Autodesk Fusion 360 part; units mm, degrees
sketch "Sketch1" plane through (0, 0, 0) normal (0, 1, 0) x (1, 0, 0)
  line L0 (0, 0) -> (-85, 0)
  line L1 (0, 0) -> (0, -98)
  line L2 (-85, 0) -> (-85, -20)
  line L3 (-85, -20) -> (-73, -20)
  line L4 (-73, -20) -> (-73, -68)
  line L5 (-73, -68) -> (-50, -98)
  line L6 (-50, -98) -> (0, -98)
  line L7 (50, -98) -> (0, -98)
  line L8 (73, -68) -> (50, -98)
  line L9 (73, -20) -> (73, -68)
  line L10 (85, -20) -> (73, -20)
  line L11 (85, 0) -> (85, -20)
  line L12 (0, 0) -> (85, 0)
  dimension "d1" = 85
  dimension "d2" = 20
  dimension "d3" = 12
  dimension "d4" = 48
  dimension "d5" = 98
  dimension "d6" = 50
extrude "Extrude1" add sketch "Sketch1" along normal blind 10
sketch "Sketch2" plane through (0, 10, 0) normal (0, 1, 0) x (-1, 0, 0)
  line L0 (85, 0) -> (85, 20)
  line L1 (85, 20) -> (73, 20)
  line L2 (73, 20) -> (73, 68)
  line L3 (73, 68) -> (50, 98)
  line L4 (50, 98) -> (-50, 98)
  line L5 (-50, 98) -> (-73, 68)
  line L6 (-73, 68) -> (-73, 20)
  line L7 (-73, 20) -> (-85, 20)
  line L8 (-85, 20) -> (-85, 0)
  line L9 (-85, 0) -> (85, 0)
  line L10 (-63, 0) -> (-63, 64.6078)
  line L11 (-63, 64.6078) -> (-37.3993, 98)
  line L12 (0, 98) -> (0, 0)
  line L13 (63, 64.6078) -> (37.3993, 98)
  line L14 (63, 0) -> (63, 64.6078)
  dimension "d9" = 10
  dimension "d10" = 10
extrude "Extrude2" add sketch "Sketch2" along normal blind 21.5 contours L4 L9 L12 L13 L14 | L4 L9 L10 L11 L12
sketch "Sketch3" plane through (0, 10, 0) normal (0, 1, 0) x (-1, 0, 0)
  line L0 (-63, 64.6078) -> (-37.3993, 98)
  line L1 (-37.3993, 98) -> (-50, 98)
  line L2 (-50, 98) -> (-73, 68)
  line L3 (-73, 68) -> (-73, 20)
  line L4 (-73, 20) -> (-85, 20)
  line L5 (-85, 20) -> (-85, 0)
  line L6 (-85, 0) -> (-63, 0)
  line L7 (-63, 0) -> (-63, 64.6078)
  line L8 (-73, 20) -> (-85, 20)
  line L9 (-85, 20) -> (-85, 0)
  line L10 (-85, 0) -> (-73, 0)
  line L11 (-73, 0) -> (-73, 20)
  line L12 (0, 0) -> (0, 105.5931)
  line L13 (73, 20) -> (85, 20)
  line L14 (73, 0) -> (73, 20)
  line L15 (85, 20) -> (85, 0)
  line L16 (85, 0) -> (73, 0)
  line L17 (-68.17, 74.3) -> (-60.2339, 68.2157)
  line L18 (-60.2339, 68.2157) -> (-63, 64.6078)
  line L19 (-63, 60) -> (-73, 60)
  line L20 (-73, 68) -> (-68.17, 74.3)
  line L21 (-73, 68) -> (-73, 60)
  line L22 (-63, 60) -> (-63, 64.6078)
  line L23 (63, 60) -> (73, 60)
  line L24 (63, 60) -> (63, 64.6078)
  line L25 (60.2339, 68.2157) -> (63, 64.6078)
  line L26 (68.17, 74.3) -> (60.2339, 68.2157)
  line L27 (73, 68) -> (68.17, 74.3)
  line L28 (73, 68) -> (73, 60)
  dimension "d15" = 8
  dimension "d20" = 6.3
extrude "Extrude3" cut sketch "Sketch3" against normal blind 6.5 contours L0 L2 L3 L7 L17 L18 L19 L20 L21 L22 | L4 L5 L6 L8 L9 L10 L11 | L13 L14 L15 L16 | L23 L24 L25 L26 L27 L28
equation "d1 = ( 170 / 2 ) * 1 mm"
equation "d10 = d9"
CAD build for the part. Positions are in the model's coordinates, mm. A direction names the side the tool comes from. Round coordinates to 2 decimals unless told otherwise and drop trailing zeros. Order: outer loops, then holes, each group sorted by start corner. A loop starts at its lowest first (then second) coordinate and runs counter-clockwise, first axis right, second up. Notation, with made-up numbers: (2, -30.5) -> (11, -30.5) arc R24 ccw to (11, -11.5) -> close; hole circle Ø6 at (80, -39). An arc over 180 degrees is marked (long way). One line per question, with ' | ' between items.
Q1. Drop flat-ended pins along their axis: pin 1 (5 mm diameter, centred on y = 16.5, z = 34.5, fed in from +X); pin 2 (8.5 mm diameter, centred on y = 16.5, z = 24, fed in from -X); pin 3 (10 mm diameter, centred on x = -66, z = 69.5, fed in from +Y). Give the stop position or say it passes through.
Completed:
pin 1: stops at x = 63 | pin 2: stops at x = -63 | pin 3: stops at y = 10
Q2. Two-plate mould, pull along Z, no slides. Class faces 6 (the flat face through (1, 16, 0)), 7 (the flat face through (-59.11, 4.93, 86.12)), 8 (the flat face through (-64.26, 6.8, 71.3)), 9 (the flat face through (68, 3.5, 66)): released by +Z, released by -Z, zero draft, split by the parting line, or undercut.
Completed:
face 6: released by -Z | face 7: released by +Z | face 8: undercut | face 9: undercut
Q3. Slice it at D-D (z = 16.5). Write the cut outline in (x, y), then the cut area to 3 significant figures.
Completed:
outline: (-85, 0) -> (85, 0) -> (85, 3.5) -> (73, 3.5) -> (73, 10) -> (63, 10) -> (63, 31.5) -> (-63, 31.5) -> (-63, 10) -> (-73, 10) -> (-73, 3.5) -> (-85, 3.5) -> close | area: 4,250 mm^2
Q4. Slice it at A-A (z = 45). Write the cut outline in (x, y), then the cut area to 3 significant figures.
Completed:
outline: (-73, 0) -> (73, 0) -> (73, 10) -> (63, 10) -> (63, 31.5) -> (-63, 31.5) -> (-63, 10) -> (-73, 10) -> close | area: 4,170 mm^2
Q5. Slice it at C-C (x = -58.5). Write the cut outline in (y, z), then the cut area to 3 significant figures.
Completed:
outline: (0, 0) -> (31.5, 0) -> (31.5, 70.48) -> (10, 70.48) -> (10, 86.91) -> (0, 86.91) -> close | area: 2,380 mm^2
Q6. Probe probe 1 along Y at (x, z) = (-68, 6.5); probe 2 along X at (y, z) = (14, 41); probe 3 along X at (y, z) = (7.5, 21.5). List the from-to ranges inside material, lowest first.
Completed:
probe 1: y = 0 to 10 | probe 2: x = -63 to 63 | probe 3: x = -73 to 73
Q7. Which spindle directions (+Z, -Z, +X, -X, +Y, -Y) get a long thin tool onto all of the face, cutting with end or side? Do faces 1 (the flat face through (-79, 2, 20)), 2 (the flat face through (79, 2, 20)), 3 (the flat face through (-79, 3.5, 10)), 4 (the flat face through (79, 3.5, 10)), 5 (the flat face through (64.26, 6.8, 71.3)). Say none if no direction does.
Completed:
face 1: +Z, -X, +Y, -Y | face 2: +Z, +X, +Y, -Y | face 3: +Z, -Z, -X, +Y | face 4: +Z, -Z, +X, +Y | face 5: +X, +Y
Q8. Slice it at B-B (y = 24). Write the cut outline in (x, z), then the cut area to 3 significant figures.
Completed:
outline: (-63, 0) -> (63, 0) -> (63, 64.61) -> (37.4, 98) -> (-37.4, 98) -> (-63, 64.61) -> close | area: 11,500 mm^2
